The listing builds one solid part. Answer for the finished solid, in the listing's coordinates (mm). A direction names the side the tool comes from. Round coordinates to 2 decimals unless told otherwise and drop trailing zeros. Write each loop counter-clockwise with the first axis right and the second up, starting at its lowest first coordinate (ties: lowest second). Pieces come first, ordered by that corner, then holes.
from build123d import *

# Parameters (mm, degrees)
BOSS_EXTRUDE1_DEPTH = 300
SKETCH2_R           = 3.75
CUT_EXTRUDE1_DEPTH  = 5.3
SKETCH3_R           = 2.25
CUT_EXTRUDE2_DEPTH  = 301.46838436


with BuildPart() as part:
    # Sketch1 → Boss-Extrude1 (new body)
    with BuildSketch(Plane.XY):
        Polygon((-7.5, 0), (7.5, 0), (7.5, 4), (5.5, 6), (5.5, 9), (7.5, 11), (7.5, 15), (-7.5, 15), (-7.5, 11), (-5.5, 9), (-5.5, 6), (-7.5, 4), align=None)
    extrude(amount=BOSS_EXTRUDE1_DEPTH)

    # Sketch2 → Cut-Extrude1 (cut)
    with BuildSketch(Plane(origin=(0, 15, 0), x_dir=(1, 0, 0), z_dir=(0, 1, 0))):
        with Locations(Location((0, -20, 0), (0, 0, 270))):
            Circle(SKETCH2_R)
        with Locations(Location((0, -80, 0), (0, 0, 270))):
            Circle(SKETCH2_R)
        with Locations(Location((0, -140, 0), (0, 0, 270))):
            Circle(SKETCH2_R)
        with Locations(Location((0, -200, 0), (0, 0, 270))):
            Circle(SKETCH2_R)
        with Locations(Location((0, -260, 0), (0, 0, 270))):
            Circle(SKETCH2_R)
    extrude(amount=-CUT_EXTRUDE1_DEPTH, mode=Mode.SUBTRACT)

    # Sketch3 → Cut-Extrude2 (cut, through all)
    with BuildSketch(Plane(origin=(0, 15, 0), x_dir=(1, 0, 0), z_dir=(0, 1, 0))):
        with Locations(Location((0, -20, 0), (0, 0, 270))):
            Circle(SKETCH3_R)
        with Locations(Location((0, -80, 0), (0, 0, 270))):
            Circle(SKETCH3_R)
        with Locations(Location((0, -140, 0), (0, 0, 270))):
            Circle(SKETCH3_R)
        with Locations(Location((0, -200, 0), (0, 0, 270))):
            Circle(SKETCH3_R)
        with Locations(Location((0, -260, 0), (0, 0, 270))):
            Circle(SKETCH3_R)
    extrude(amount=-CUT_EXTRUDE2_DEPTH, mode=Mode.SUBTRACT)


solid = part.part
1. Section A-A on z = 103 is taken. Determine the outline of the cut face in (x, y), plus the area to 3 significant figures.
Geometry says:
outline: (-7.5, 0) - (7.5, 0) - (7.5, 4) - (5.5, 6) - (5.5, 9) - (7.5, 11) - (7.5, 15) - (-7.5, 15) - (-7.5, 11) - (-5.5, 9) - (-5.5, 6) - (-7.5, 4) - close
area: 205 mm2
2. Section B-B on x = 0 is taken. Give the number of separate pieces and of enclosed holes in the cut face, plus the area to 3 significant figures.
Geometry says:
separate pieces: 6
enclosed holes: 0
area: 4,080 mm2
3. A tool of negligible diameter and unlimited length cuts with its end or side. For faces 1 (the face through (1.126, 12.387, 263.577)), 2 (the face through (0, 0, 148)), from which of +Z, -Z, +X, -X, +Y, -Y can it reach the whole face along a straight path? Write none if from no direction.
Geometry says:
face 1: +Y
face 2: +Z, -Z, +X, -X, -Y
4. Straight lines are drawn through the part: line 1 along Z through (x, y) = (0.75, 2); line 2 along X through (y, z) = (2.75, 200); line 3 along Z through (x, y) = (-0.75, 11.5). For each, find the intervals that lie inside material, in ascending order.
Geometry says:
line 1: z = 0 to 17.88, 22.12 to 77.88, 82.12 to 137.88, 142.12 to 197.88, 202.12 to 257.88, 262.12 to 300
line 2: x = -7.5 to -2.25, 2.25 to 7.5
line 3: z = 0 to 16.33, 23.67 to 76.33, 83.67 to 136.33, 143.67 to 196.33, 203.67 to 256.33, 263.67 to 300
5. For a pull along X with two mould halves and no side action, classify faces 3 (the face through (-2, 9.7, 262)), 4 (the face through (0, 15, 148)), 5 (the face through (-2, 9.7, 22)) as released by +X, released by -X, zero draft, split by the parting line, or undercut.
Geometry says:
face 3: undercut
face 4: zero draft
face 5: undercut
6. Given pin 1 (7 mm diameter, centred on x = 0, z = 200, fed in from +Y); pin 2 (0.9 mm diameter, centred on y = 7.5, z = 224.5, fed in from +X); pin 3 (1.5 mm diameter, centred on y = 5, z = 45.5, fed in from -X), each flat-ended and moving along its own axis, determine where each tip first touches the part or whether it passes through.
Geometry says:
pin 1: stops at y = 9.7
pin 2: stops at x = 5.5
pin 3: stops at x = -7.25
